For this review, take the finished solid that the model builds, in its own axes (mm). A direction names the side the tool comes from. Give positions to 0.01 mm unless a question says otherwise; leave off trailing zeros. Loops run counter-clockwise (first coordinate to the right, second up) from the corner with the lowest first, then second, coordinate; pieces in that order, holes last. Notation, with made-up numbers: (3, 43) - (15, 43) arc R4 cw to (15, 47) - close; hole circle Ø7 at (-34, 81.5). An arc over 180 degrees is marked (long way). Put each result on its own line as item: value. Start each with the question number.
from build123d import *

# Parameters (mm, degrees)
F0_W     = 38.1
F0_H     = 23.368
F1_DEPTH = 25.4
F2_R     = 6.35
F3_DEPTH = 12.7
F4_R     = 3.175
F5_DEPTH = 25.4
F6_R     = 5.08
F8_DEPTH = 25.4


with BuildPart() as f1:
    # F0 (on Top) → F1 (new body)
    with BuildSketch(Plane.XY):
        with Locations((19.05, 11.684)):
            Rectangle(F0_W, F0_H)
    extrude(amount=F1_DEPTH)

    # F2 (on face) → F3 (cut)
    with BuildSketch(Plane.XY.offset(25.4)):
        with Locations((19.05, 11.684)):
            Circle(F2_R)
    extrude(amount=-F3_DEPTH, mode=Mode.SUBTRACT)

    # F4 (on face) → F5 (cut)
    with BuildSketch(Plane.XY.offset(12.7)):
        with Locations((19.05, 11.684)):
            Circle(F4_R)
    extrude(amount=-F5_DEPTH, mode=Mode.SUBTRACT)

    # F6
    f6_edges = [f1.edges().sort_by_distance(p)[0] for p in [
        (0, 23.368, 12.7),
        (0, 0, 12.7),
    ]]
    fillet(f6_edges, radius=F6_R)

    # F7 (on face) → F8 (cut)
    with BuildSketch(Plane(origin=(0, 23.368, 0), x_dir=(-1, 0, 0), z_dir=(0, 1, 0))):
        with BuildLine():
            Line((-38.1, 18.349398), (-38.1, 7.316839))
            ThreePointArc((-38.1, 7.316839), (-33.818122, 12.833118), (-38.1, 18.349398))
        make_face()
    extrude(amount=-F8_DEPTH, mode=Mode.SUBTRACT)


solid = f1.part
1) Mouldability with a two-part tool opening along X and no side actions: class faces 1 (the cylindrical face through (1.449, 1.528, 12.878)), 2 (the flat face through (23, 17, 25.4)), 3 (the cylindrical face through (24.916, 9.252, 19.139)) as released by +X, released by -X, zero draft, split by the parting line, or undercut.
2) Take a section at D-D on x = 15. State the section outline as (y, z) points, and give its area (3 significant figures).
3) Take a section at C-C on z = 23.5. State the section outline as (x, y) points.
4) Wall thickness on probe 1 along Y at (x, z) = (19.05, 8); probe 2 along Y at (x, z) = (19.05, 19); probe 3 along X at (y, z) = (11.5, 7): over which ranges is each line inside the solid? List them lowest first.
5) Take a section at A-A on x = 19.05. State the section outline as (y, z) points, and give its area (3 significant figures).
6) Machinability: for faces 4 (the flat face through (21, 0, 13)), 5 (the flat face through (20, 15, 12.7)), which of the approach directions +Z, -Z, +X, -X, +Y, -Y give a long, thin tool a straight path to every point of the face, cutting with its end or side? Answer none if there is none.
7) Insertion check: P1, Ø10, axis at x = 19.5, y = 14, coming from the +Z side. The pin has a flat end and moves straight along its axis. Give the tip position at first contact, or say it passes through.
8) Take a section at B-B on y = 14. State the section outline as (x, z) points.
Answers follow:
1. face 1: released by -X
1. face 2: zero draft
1. face 3: undercut
2. outline: (0, 0) - (23.37, 0) - (23.37, 25.4) - (16.57, 25.4) - (16.57, 12.7) - (6.79, 12.7) - (6.79, 25.4) - (0, 25.4) - close
2. area: 469 mm2
3. outline: (0, 5.08) arc R5.08 ccw to (5.08, 0) - (38.1, 0) - (38.1, 23.37) - (5.08, 23.37) arc R5.08 ccw to (0, 18.29) - close; hole circle Ø12.7 at (19.05, 11.68)
4. probe 1: 0 to 8.51, 14.86 to 23.37
4. probe 2: 0 to 5.33, 18.03 to 23.37
4. probe 3: 0 to 15.88, 22.22 to 38.1
5. outline: (0, 0) - (8.51, 0) - (8.51, 12.7) - (5.33, 12.7) - (5.33, 25.4) - (0, 25.4) - close; (14.86, 0) - (23.37, 0) - (23.37, 25.4) - (18.03, 25.4) - (18.03, 12.7) - (14.86, 12.7) - close
5. area: 352 mm2
6. face 4: +Z, -Z, +X, -X, -Y
6. face 5: +Z
7. P1: z = 25.4
8. outline: (0, 0) - (16.88, 0) - (16.88, 12.7) - (13.14, 12.7) - (13.14, 25.4) - (0, 25.4) - close; (21.22, 0) - (38.1, 0) - (38.1, 7.32) arc R5.69 cw to (38.1, 18.35) - (38.1, 25.4) - (24.96, 25.4) - (24.96, 12.7) - (21.22, 12.7) - close
